```python
from build123d import *

# Parameters (mm, degrees)
SKETCH1_W          = 41.148
SKETCH1_H          = 18.0848
SKETCH1_W_2        = 19.431
SKETCH1_H_2        = 13.081
EXTRUDE1_DEPTH     = 17.4498
SKETCH2_W          = 8.3566
SKETCH2_H          = 18.0848
CUT_EXTRUDE1_DEPTH = 14.2748
CUT_EXTRUDE2_START = -1.5748
SKETCH3_W          = 24.4348
SKETCH3_H          = 18.0848
SKETCH3_W_2        = 21.4376
SKETCH3_H_2        = 14.5796
CUT_EXTRUDE2_DEPTH = 12.7
SKETCH4_R          = 1.6383
CUT_EXTRUDE3_DEPTH = 4.175
CHAMFER1_SIZE      = 0.508
FILLET1_R          = 0.254
CHAMFER2_SIZE      = 0.508


with BuildPart() as part:
    # Sketch1 → Extrude1 (new body)
    with BuildSketch(Plane(origin=(0, 0, 0), x_dir=(1, 0, 0), z_dir=(0, 1, 0))):
        with Locations((20.574, 9.0424)):
            Rectangle(SKETCH1_W, SKETCH1_H)
        with Locations((20.574, 9.0424)):
            Rectangle(SKETCH1_W_2, SKETCH1_H_2, mode=Mode.SUBTRACT)
    extrude(amount=EXTRUDE1_DEPTH)

    # Sketch2 → Cut-Extrude1 (cut)
    with BuildSketch(Plane(origin=(0, 17.4498, 0), x_dir=(-1, 0, 0), z_dir=(0, 1, 0))):
        with Locations((-4.1783, -9.0424)):
            Rectangle(SKETCH2_W, SKETCH2_H)
        with Locations((-36.9697, -9.0424)):
            Rectangle(SKETCH2_W, SKETCH2_H)
    extrude(amount=-CUT_EXTRUDE1_DEPTH, mode=Mode.SUBTRACT)

    # Sketch3 → Cut-Extrude2 (cut)
    with BuildSketch(Plane(origin=(0, 17.4498, 0), x_dir=(-1, 0, 0), z_dir=(0, 1, 0)).offset(CUT_EXTRUDE2_START)):
        with Locations((-20.574, -9.0424)):
            Rectangle(SKETCH3_W, SKETCH3_H)
        with Locations((-20.574, -9.0424)):
            Rectangle(SKETCH3_W_2, SKETCH3_H_2, mode=Mode.SUBTRACT)
    extrude(amount=-CUT_EXTRUDE2_DEPTH, mode=Mode.SUBTRACT)

    # Sketch4 → Cut-Extrude3 (cut, through all)
    with BuildSketch(Plane(origin=(0, 3.175, 0), x_dir=(-1, 0, 0), z_dir=(0, 1, 0))):
        with Locations(Location((-36.4998, -13.7922, 0), (0, 0, 90))):  # turned: the seam where the file's is
            Circle(SKETCH4_R)
        with Locations(Location((-36.4998, -4.2672, 0), (0, 0, 90))):  # turned: the seam where the file's is
            Circle(SKETCH4_R)
        with Locations(Location((-4.6482, -4.2672, 0), (0, 0, 90))):  # turned: the seam where the file's is
            Circle(SKETCH4_R)
        with Locations(Location((-4.6482, -13.7922, 0), (0, 0, 90))):  # turned: the seam where the file's is
            Circle(SKETCH4_R)
    extrude(amount=-CUT_EXTRUDE3_DEPTH, mode=Mode.SUBTRACT)

    # Chamfer1
    chamfer1_edges = [part.edges().sort_by_distance(p)[0] for p in [
        (36.4998, 3.175, -15.4305),
        (36.4998, 3.175, -5.9055),
        (4.6482, 3.175, -5.9055),
        (4.6482, 3.175, -15.4305),
    ]]
    chamfer(chamfer1_edges, length=CHAMFER1_SIZE)

    # Fillet1
    fillet1_edges = [part.edges().sort_by_distance(p)[0] for p in [
        (10.8585, 8.7249, -15.5829),
        (10.8585, 8.7249, -2.5019),
        (30.2895, 8.7249, -2.5019),
        (30.2895, 8.7249, -15.5829),
    ]]
    fillet(fillet1_edges, radius=FILLET1_R)

    # Chamfer2
    chamfer2_edges = [part.edges().sort_by_distance(p)[0] for p in [
        (36.4998, 0, -15.4305),
        (36.4998, 0, -5.9055),
        (4.6482, 0, -5.9055),
        (4.6482, 0, -15.4305),
    ]]
    chamfer(chamfer2_edges, length=CHAMFER2_SIZE)


solid = part.part
```
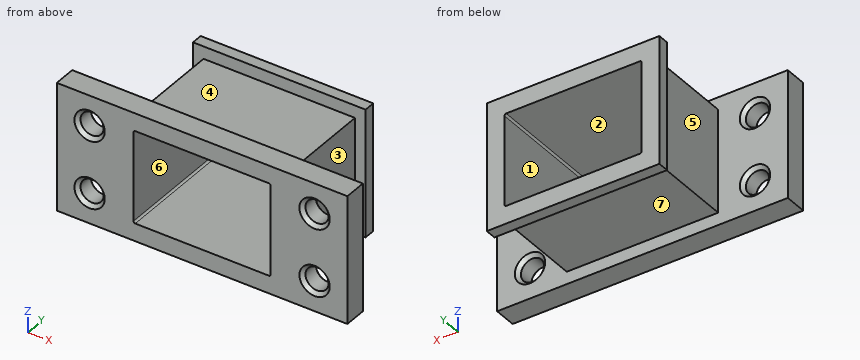
Geometry: final body of the model. Coordinates: model frame, mm. Face numbers are marked on the shaded views. A direction names the side the tool comes from. Coordinates: 2 decimals unless noted, no trailing zeros. Order: outer loops, then holes, each group sorted by start corner. A loop starts at its lowest first (then second) coordinate and runs counter-clockwise, first axis right, second up. Notation, with made-up numbers: (34, 87) - (92, 87) arc R24 ccw to (92, 100) - close; hole circle Ø3 at (14, 3.5). An arc over 180 degrees is marked (long way). Write each question's results on one line, items separated by ' | '.
(1) Set-up query: the marked faces 5, 6 and 7. Return all of +Z, -Z, +X, -X, +Y, -Y with unobstructed straight access to the full face (end or side cutting, diameter ignored); none if empty.
Values found:
face 5: +Z, -Z, -X | face 6: +Y, -Y | face 7: -Z, +X, -X
(2) Line query: line 1 (Z direction, x = 26.5, y = 1.75); line 2 (Z direction, x = 14.5, y = 13.75); line 3 (X direction, y = 4, z = -4). Output: solid intervals per line, ascending. Write a range as [from, to].
Values found:
line 1: z = [-18.08, -15.58], [-2.5, 0] | line 2: z = [-16.33, -15.58], [-2.5, -1.75] | line 3: x = [9.86, 10.86], [30.29, 31.29]
(3) Section query C-C, the plane y = 16.5. Return the cut outline in (x, z), plus the area to 3 significant figures.
Values found:
outline: (8.36, -18.08) - (32.79, -18.08) - (32.79, 0) - (8.36, 0) - close; hole (10.86, -15.33) arc R0.25 ccw to (11.11, -15.58) - (30.04, -15.58) arc R0.25 ccw to (30.29, -15.33) - (30.29, -2.76) arc R0.25 ccw to (30.04, -2.5) - (11.11, -2.5) arc R0.25 ccw to (10.86, -2.76) - close | area: 188 mm²
(4) First-contact query: pin 1 Ø1 at (y, z) = (12, -6.5) entering from +X; pin 2 Ø1.7 at (y, z) = (16.5, -8) entering from -X; pin 3 Ø1.5 at (x, y) = (29.5, 7) entering from -Z. Flat tips, straight axial feed; report the tip coordinate or a pass-through.
Values found:
pin 1: stops at x = 31.29 | pin 2: stops at x = 8.36 | pin 3: stops at z = -16.33
(5) Section query D-D, the plane y = 12.5. Return the cut outline in (x, z).
Values found:
outline: (9.86, -16.33) - (31.29, -16.33) - (31.29, -1.75) - (9.86, -1.75) - close; hole (10.86, -15.33) arc R0.25 ccw to (11.11, -15.58) - (30.04, -15.58) arc R0.25 ccw to (30.29, -15.33) - (30.29, -2.76) arc R0.25 ccw to (30.04, -2.5) - (11.11, -2.5) arc R0.25 ccw to (10.86, -2.76) - close
(6) Mould query, pull axis Z, two halves, no side actions, for the marked faces 1, 2, 3 and 4. Classes: +Z half, -Z half, draft (parallel to the pull), parting line (faces both ways), or undercut.
Values found:
face 1: undercut | face 2: undercut | face 3: draft | face 4: +Z half
(7) Section query A-A, the plane z = -10.5. Return the cut outline in (x, y) (1 decimal).
Values found:
outline: (0, 0) - (10.9, 0) - (10.9, 17.4) - (8.4, 17.4) - (8.4, 15.9) - (9.9, 15.9) - (9.9, 3.2) - (0, 3.2) - close; (30.3, 0) - (41.1, 0) - (41.1, 3.2) - (31.3, 3.2) - (31.3, 15.9) - (32.8, 15.9) - (32.8, 17.4) - (30.3, 17.4) - close
(8) Section query B-B, the plane x = 12. Return the cut outline in (y, z) (3 decimals).
Values found:
outline: (0, -18.085) - (3.175, -18.085) - (3.175, -16.332) - (15.875, -16.332) - (15.875, -18.085) - (17.45, -18.085) - (17.45, -15.583) - (0, -15.583) - close; (0, -2.502) - (17.45, -2.502) - (17.45, 0) - (15.875, 0) - (15.875, -1.753) - (3.175, -1.753) - (3.175, 0) - (0, 0) - close
